```python
from build123d import *

# Parameters (mm, degrees)
SKETCH1_R           = 20
BOSS_EXTRUDE1_DEPTH = 200
SKETCH2_R           = 30
BOSS_EXTRUDE2_DEPTH = 15
SKETCH3_W           = 34
SKETCH3_H           = 40
BOSS_EXTRUDE3_DEPTH = 30
CUT_EXTRUDE1_DEPTH  = 59
FILLET1_R           = 15
SKETCH5_R           = 5
CUT_EXTRUDE2_DEPTH  = 59


with BuildPart() as part:
    # Sketch1 → Boss-Extrude1 (new body)
    with BuildSketch(Plane(origin=(0, 0, 0), x_dir=(1, 0, 0), z_dir=(0, 1, 0))):
        with Locations(Location((0, 0, 0), (0, 0, 270))):
            Circle(SKETCH1_R)
    extrude(amount=BOSS_EXTRUDE1_DEPTH)

    # Sketch2 → Boss-Extrude2 (add)
    with BuildSketch(Plane(origin=(0, 200, 0), x_dir=(1, 0, 0), z_dir=(0, 1, 0))):
        with Locations(Location((0, 0, 0), (0, 0, 270))):
            Circle(SKETCH2_R)
    extrude(amount=BOSS_EXTRUDE2_DEPTH)

    # Sketch3 → Boss-Extrude3 (add)
    with BuildSketch(Plane(origin=(0, 215, 0), x_dir=(1, 0, 0), z_dir=(0, 1, 0))):
        Rectangle(SKETCH3_W, SKETCH3_H)
    extrude(amount=BOSS_EXTRUDE3_DEPTH)

    # Sketch4 → Cut-Extrude1 (cut)
    with BuildSketch(Plane(origin=(17, 0, 0), x_dir=(0, 0, -1), z_dir=(1, 0, 0))):
        Polygon((20, 215), (-5, 245), (20, 245), align=None)
    extrude(amount=-CUT_EXTRUDE1_DEPTH, mode=Mode.SUBTRACT)

    # Fillet1
    fillet1_edges = [part.edges().sort_by_distance(p)[0] for p in [
        (0, 245, 20),
    ]]
    fillet(fillet1_edges, radius=FILLET1_R - 0.0001)  # a hair under: the kernel refuses the full size

    # Sketch5 → Cut-Extrude2 (cut)
    with BuildSketch(Plane(origin=(17, 0, 0), x_dir=(0, 0, -1), z_dir=(1, 0, 0))):
        with Locations((-9.891874818, 235.24975043)):
            Circle(SKETCH5_R)
    extrude(amount=-CUT_EXTRUDE2_DEPTH, mode=Mode.SUBTRACT)


solid = part.part
```
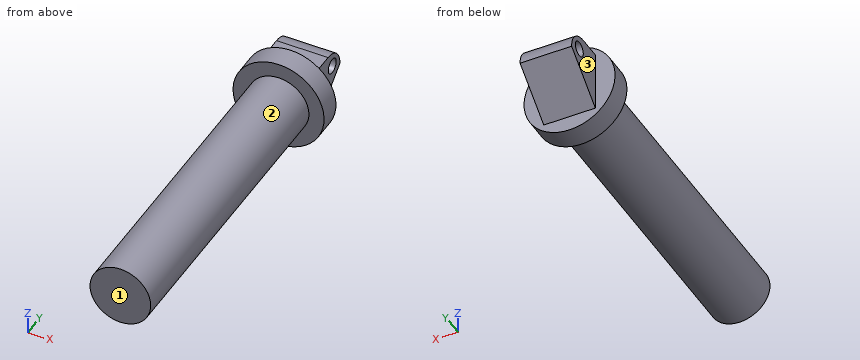
Input: part model. Units: mm. Frame: model coordinates. Face numbers are marked on the shaded views. A direction names the side the tool comes from. Coordinates: 2 decimals unless noted, no trailing zeros. Loops run counter-clockwise (first coordinate to the right, second up) from the corner with the lowest first, then second, coordinate; pieces in that order, holes last. Notation, with made-up numbers: M 14.5,-1 L 39.5,-1 A25 ccw 39.5,33 Z; hole C 16.25,89.25 d2. An arc over 180 degrees is marked long. One line per item, written item: value.
(1) Section B-B (z = 0). Output: boundary loops of the cut face in (x, y), and give its area (3 significant figures).
Filled in:
outline: M -30,200 L -20,200 L -20,0 L 20,0 L 20,200 L 30,200 L 30,215 L 17,215 L 17,239 L -17,239 L -17,215 L -30,215 Z
area: 9,720 mm^2
(2) Pin query (flat end, axial travel): pin 1 (6 mm diameter, centred on x = -14.5, y = 100.5, fed in from -Z); pin 2 (1.5 mm diameter, centred on x = -16, y = 101.5, fed in from -Z); pin 3 (5 mm diameter, centred on y = 105.5, z = -8, fed in from -X); pin 4 (3 mm diameter, centred on x = 9.5, z = 3.5, fed in from -Y). Return the tip coordinate at first contact, or that it passes through.
Filled in:
pin 1: z = -16.36
pin 2: z = -12.94
pin 3: x = -19.23
pin 4: y = 0
(3) Reachability of the marked faces 1, 2 and 3 from +Z, -Z, +X, -X, +Y, -Y: full face, straight path, thin tool, end or side. Return the list, or none.
Filled in:
face 1: +Z, -Z, +X, -X, -Y
face 2: -Y
face 3: +Z, -Z, -X, +Y
(4) Section D-D (x = 23). Output: boundary loops of the cut face in (y, z).
Filled in:
outline: M 200,-19.26 L 215,-19.26 L 215,19.26 L 200,19.26 Z
(5) Line query: line 1 along Y through (x, z) = (-10.5, -23.5); line 2 along X through (y, z) = (40.5, 0); line 3 along X through (y, z) = (222, 3). Output: solid intervals per line, ascending. Write a range as from..to.
Filled in:
line 1: 200..215
line 2: -20..20
line 3: -17..17
(6) Section C-C (y = 103). Output: boundary loops of the cut face in (x, z), and give its area (3 significant figures).
Filled in:
outline: C 0,0 d40
area: 1,260 mm^2
